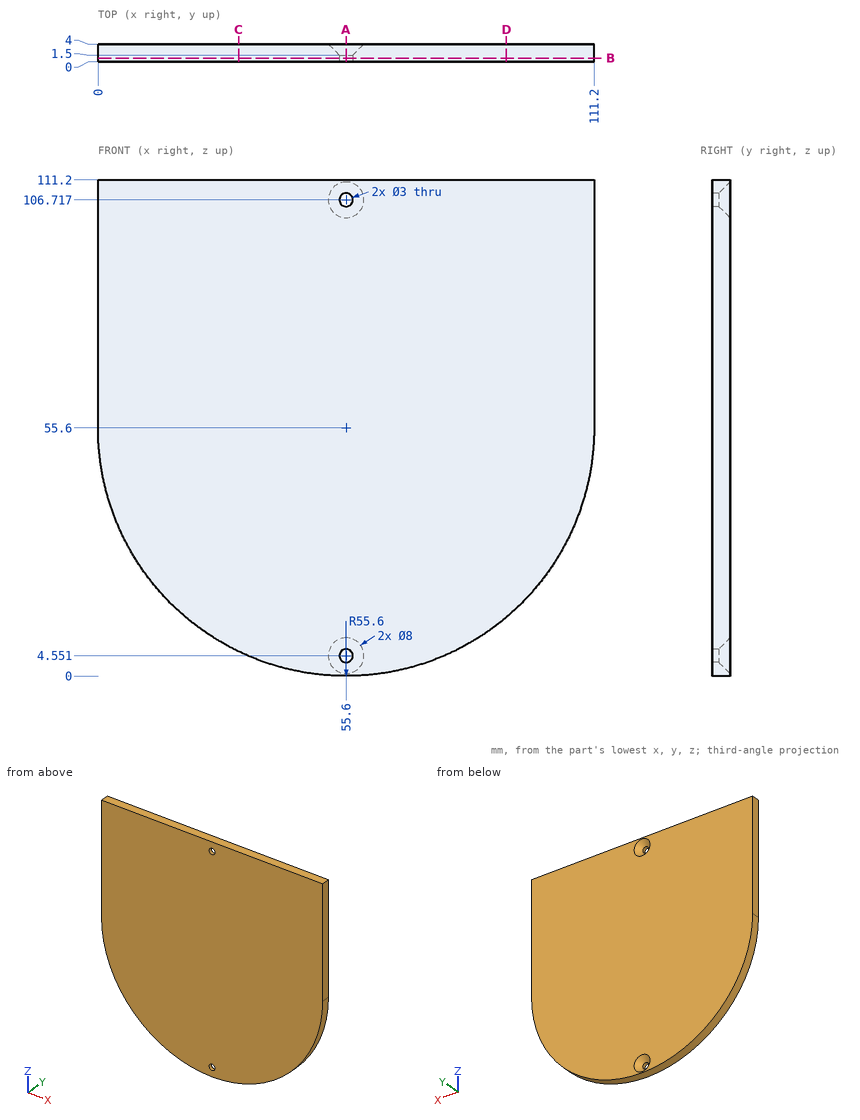
For this review, use the dimensioned drawing (mm, ordinates from the lowest corner) and the shaded views. Coordinates: 2 decimals unless noted, no trailing zeros. Write each loop counter-clockwise with the first axis right and the second up, starting at its lowest first coordinate (ties: lowest second). Pieces come first, ordered by that corner, then holes. Notation, with made-up numbers: (65.5, 29.5) -> (85.5, 29.5) arc R11 ccw to (85.5, 33.5) -> close; hole circle Ø8 at (-10.75, 43.5). An arc over 180 degrees is marked (long way). Put each result on its own line as item: value.
Q1. Wall thickness on L1, parallel to Z at x = 55.6, y = 0.9; L2, parallel to Z at x = 54, y = 3.85; L3, parallel to Z at x = 98, y = 1.2: over which ranges is each line inside the solid? List them lowest first.
From the geometry:
L1: z = 0 to 3.05, 6.05 to 105.22, 108.22 to 111.2
L2: z = 0.02 to 1.05, 8.05 to 103.22, 110.22 to 111.2
L3: z = 19.63 to 111.2
Q2. Take a section at A-A, the plane x = 55.6. State the section outline as (y, z) points, then the cut area to 3 significant figures.
From the geometry:
outline: (0, 0) -> (4, 0) -> (4, 0.55) -> (1.5, 3.05) -> (0, 3.05) -> close; (0, 6.05) -> (1.5, 6.05) -> (4, 8.55) -> (4, 102.72) -> (1.5, 105.22) -> (0, 105.22) -> close; (0, 108.22) -> (1.5, 108.22) -> (4, 110.72) -> (4, 111.2) -> (0, 111.2) -> close
area: 408 mm2
Q3. Take a section at D-D, the plane x = 91.5. State the section outline as (y, z) points.
From the geometry:
outline: (0, 13.14) -> (4, 13.14) -> (4, 111.2) -> (0, 111.2) -> close
Q4. Take a section at B-B, the plane y = 0.85. State the section outline as (x, z) points.
From the geometry:
outline: (0, 55.6) arc R55.6 ccw to (111.2, 55.6) -> (111.2, 111.2) -> (0, 111.2) -> close; hole circle Ø3 at (55.6, 4.55); hole circle Ø3 at (55.6, 106.72)
Q5. Take a section at C-C, the plane x = 31.5. State the section outline as (y, z) points.
From the geometry:
outline: (0, 5.49) -> (4, 5.49) -> (4, 111.2) -> (0, 111.2) -> close
Q6. Clearance check with flat-ended pins moving along their axes: pin 1 Ø1.5 at (y, z) = (2, 14.5) entering from -X; pin 2 Ø1.8 at (x, z) = (55.6, 106.717) entering from -Y. State where each tip first meets the part, or that it passes through.
From the geometry:
pin 1: stops at x = 17.35
pin 2: passes through
